Part model, mm, in its own coordinate system. Give positions to 0.01 mm unless a question says otherwise; leave off trailing zeros. Loops run counter-clockwise (first coordinate to the right, second up) from the corner with the lowest first, then second, coordinate; pieces in that order, holes last. Notation, with made-up numbers: M 5,-6 L 45,-6 A16 cw 45,6 Z; hole C 10,58 d1. An arc over 180 degrees is marked long. Answer in a Markdown table with one row per item.
from build123d import *

# Parameters (mm, degrees)
F0_R     = 11
F1_DEPTH = 7
F2_R     = 3.95
F3_DEPTH = 7.001
F4_R     = 0.5


with BuildPart() as f1:
    # F0 (on Top) → F1 (new body)
    with BuildSketch(Plane.XY):
        Circle(F0_R)
    extrude(amount=F1_DEPTH)

    # F2 (on face) → F3 (cut, through all)
    with BuildSketch(Plane.XY.offset(7)):
        Circle(F2_R)
    extrude(amount=-F3_DEPTH, mode=Mode.SUBTRACT)

    # F4
    f4_edges = [f1.edges().sort_by_distance(p)[0] for p in [
        (-11, 0, 7),
        (-3.95, 0, 7),
        (-11, 0, 0),
        (-3.95, 0, 0),
    ]]
    fillet(f4_edges, radius=F4_R)


solid = f1.part
(1) Saw through at A-A (y = 0). Write the cut outline in (x, z).
Recorded:
| item | result |
|---|---|
| outline | M -11,0.5 A0.5 ccw -10.5,0 L -4.45,0 A0.5 ccw -3.95,0.5 L -3.95,6.5 A0.5 ccw -4.45,7 L -10.5,7 A0.5 ccw -11,6.5 Z; M 3.95,0.5 A0.5 ccw 4.45,0 L 10.5,0 A0.5 ccw 11,0.5 L 11,6.5 A0.5 ccw 10.5,7 L 4.45,7 A0.5 ccw 3.95,6.5 Z |
(2) Pull direction Y, two halves, no side cores. Call faces 1 (the face through (-2.38, -10.74, 3.46)), 2 (the face through (5, 0, 0)), 3 (the face through (-3.135, -2.404, 3.542)): +Y half, -Y half, draft (parallel to the pull), parting line (faces both ways), or undercut.
Recorded:
| item | result |
|---|---|
| face 1 | parting line |
| face 2 | draft |
| face 3 | undercut |
(3) Pin check, flat tips, straight feed: pin 1 Ø2 at (x, z) = (-4, 3) entering from -Y; pin 2 Ø4.5 at (x, y) = (0, 0) entering from +Z; pin 3 Ø3 at (y, z) = (5.5, 5.5) entering from -X; pin 4 Ø2 at (y, z) = (-6.5, 2) entering from +X. Stop position of each tip, or through.
Recorded:
| item | result |
|---|---|
| pin 1 | stops at y = -10.58 |
| pin 2 | passes through |
| pin 3 | stops at x = -10.25 |
| pin 4 | stops at x = 9.53 |
(4) Saw through at C-C (z = 1.5). Write the cut outline in (x, y).
Recorded:
| item | result |
|---|---|
| outline | C 0,0 d22; hole C 0,0 d7.9 |
(5) Drill centre lines: line 1 along Y through (x, z) = (0, 3.8); line 2 along X through (y, z) = (-0.25, 1); line 3 along X through (y, z) = (-3, 6). Where is each one in solid material? Low to high.
Recorded:
| item | result |
|---|---|
| line 1 | y = -11 to -3.95, 3.95 to 11 |
| line 2 | x = -11 to -3.94, 3.94 to 11 |
| line 3 | x = -10.58 to -2.57, 2.57 to 10.58 |
